Design review of the part built by this model. Coordinates are the model's own, in mm. A direction names the side the tool comes from. Round coordinates to 2 decimals unless told otherwise and drop trailing zeros. Loops run counter-clockwise (first coordinate to the right, second up) from the corner with the lowest first, then second, coordinate; pieces in that order, holes last. Notation, with made-up numbers: M 17,36.25 L 34,36.25 A19 ccw 34,63.25 Z; hole C -20.5,76 d6. An arc over 180 degrees is marked long. Use a Markdown table: item, result.
Autodesk Inventor part; units mm, degrees
ref_plane "YZ Plane" through (0, 0, 0) normal (1, 0, 0) x (0, 1, 0)
ref_plane "XZ Plane" through (0, 0, 0) normal (0, 1, 0) x (-1, 0, 0)
ref_plane "XY Plane" through (0, 0, 0) normal (0, 0, 1) x (1, 0, 0)
sketch "Sketch1" plane through (0, 0, 0) normal (0, 1, 0) x (-1, 0, 0)
  circle A0 centre (0, 0) radius 2.5
  circle A1 centre (0, 0) radius 1.5
  dimension "d0" = 5
  dimension "d1" = 3
extrude "Extrusion1" add sketch "Sketch1" along normal blind 1
sketch "Sketch2" plane through (0, 1, 0) normal (0, 1, 0) x (1, 0, 0)
  circle A0 centre (0, 0) radius 1.5
  dimension "d4" = 3
extrude "Extrusion2" add sketch "Sketch2" along normal blind 5 and the other way blind 1
sketch "Sketch4" plane through (0, 0, 0) normal (0, -1, 0) x (1, 0, 0)
  circle A0 centre (0, 0) radius 1.5
  line L0 (-0.1651, 0.1041) -> (-0.1651, 1.4909)
  line L1 (0.1791, 0.0776) -> (0.1791, 1.4893)
  line L2 (-0.1651, -0.1651) -> (-0.1651, -1.4909)
  line L3 (0.1791, -0.0776) -> (0.1791, -1.4893)
  line L4 (-0.1651, -0.1651) -> (-1.4909, -0.1651)
  line L5 (0.1791, -0.1651) -> (1.4909, -0.1651)
  line L6 (-0.1651, 0.1041) -> (-1.4964, 0.1041)
  line L7 (0.1791, 0.0776) -> (1.498, 0.0776)
  circle A1 centre (0, 0) radius 0.4994
extrude "Extrusion4" cut sketch "Sketch4" against normal blind 1 contours A0 L5 A1 L7 | L1 A1 L0 A0 | A1 L5 L3 L2 L4 L6 L0 L1 L7 | L7 L1 A1 | A0 L2 A1 L3 | A1 L3 L5 | L6 A1 L4 A0 | L0 L6 A1 | A1 L4 L2
fillet "Fillet1" radius 1 1 edges at (2.5, 0, 0)
fillet "Fillet2" radius 0.2 1 edges at (-1.5, 6, 0)
sketch "Sketch5" plane through (0, 1, 0) normal (0, 1, 0) x (1, 0, 0)
  circle A0 centre (0, 0) radius 1.9093
extrude "Extrusion5" add sketch "Sketch5" along normal blind 0.1
thread "Thread1"
properties part number "screw"
1. Insertion check: pin 1 (1 mm diameter, centred on y = 2.5, z = 1.5, fed in from +X); pin 2 (0.8 mm diameter, centred on y = 0.5, z = 1, fed in from +X); pin 3 (0.5 mm diameter, centred on x = 1, y = 0.5, fed in from +Z). Each pin has a flat end and moves straight along its axis. Give the tip position at first contact, or say it passes through.
Check values:
| item | result |
|---|---|
| pin 1 | stops at x = 1.12 |
| pin 2 | stops at x = 2.37 |
| pin 3 | stops at z = 2.3 |
2. Take a section at C-C on y = 1.3. Give the boundary of the cut face in (x, z), and give its area (3 significant figures).
Check values:
| item | result |
|---|---|
| outline | C 0,0 d3 |
| area | 7.07 mm² |
3. Wall thickness on line 1 along X through (y, z) = (5, -0.1); line 2 along Z through (x, y) = (0.7, 0.65); line 3 along Z through (x, y) = (-0.3, 0.75): over which ranges is each line inside the solid? List them lowest first. Write a range as from..to.
Check values:
| item | result |
|---|---|
| line 1 | x = -1.5..1.5 |
| line 2 | z = -2.33..-0.17, 0.08..2.33 |
| line 3 | z = -2.45..-0.4, 0.4..2.45 |
4. The part is to be moulded in two halves that separate along X. For faces 1 (the face through (-1.5, 3.42, 0.07)), 2 (the face through (0.179, 0.5, -1)), 3 (the face through (-0.6, 0, 0.4)), say which applies: pulls with the +X half, pulls with the -X half, needs draft (parallel to the pull), parting line crosses it, or undercut.
Check values:
| item | result |
|---|---|
| face 1 | parting line crosses it |
| face 2 | undercut |
| face 3 | needs draft |
5. Machinability: for faces 4 (the face through (0.179, 0.5, 1)), 5 (the face through (0, 6, 0)), 6 (the face through (1, 1, -2)), which of the approach directions +Z, -Z, +X, -X, +Y, -Y give a long, thin tool a straight path to every point of the face, cutting with its end or side? Answer none if there is none.
Check values:
| item | result |
|---|---|
| face 4 | -Y |
| face 5 | +Z, -Z, +X, -X, +Y |
| face 6 | +Y |
